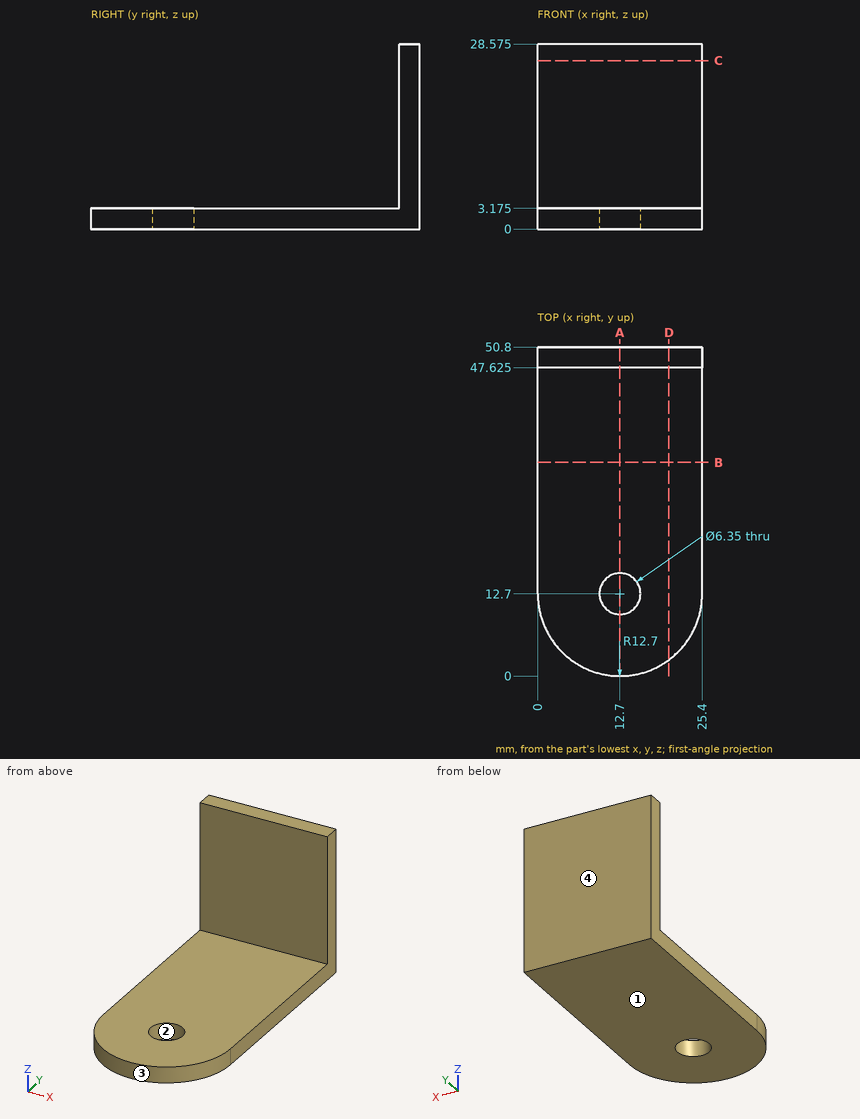
Drawing for the job (mm, zero at the part's lowest x, y, z). Round coordinates to 2 decimals unless told otherwise and drop trailing zeros. Loops run counter-clockwise (first coordinate to the right, second up) from the corner with the lowest first, then second, coordinate; pieces in that order, holes last. Notation, with made-up numbers: M 47.5,82 L 51.5,82 A27 ccw 51.5,121 Z; hole C -34,81 d7. An arc over 180 degrees is marked long. Use a Markdown table: item, result. Add a question column.
(1) Pull direction Y, two halves, no side cores. Call the marked faces 1, 2, 3 and 4: +Y half, -Y half, draft (parallel to the pull), parting line (faces both ways), or undercut.
(2) Cut at B-B (y = 33). Give the cut face in (x, z) (3 decimals), and give its area (3 significant figures).
(3) Flat gauge pins, fed straight in: pin 1 (3 mm diameter, centred on x = 7.5, y = 28, fed in from +Z) (3 decimals); pin 2 (12.5 mm diameter, centred on x = 7.5, z = 15.5, fed in from -Y) (3 decimals). Where does each tip first touch, or does it go through?
(4) Cut at C-C (z = 26). Give the cut face in (x, y) (3 decimals).
(5) Cut at A-A (x = 12.7). Give the cut face in (y, z) (3 decimals).
(6) Cut at D-D (x = 20.25). Give the cut face in (y, z) (3 decimals), and give its area (3 significant figures).
(7) Drill centre lines: line 1 (Y direction, x = 12.7, z = 2.05) (3 decimals); line 2 (Y direction, x = 18.25, z = 26) (3 decimals); line 3 (Z direction, x = 8, y = 9) (3 decimals). Where is each one in solid material? Low to high.
Geometry says:
| question | item | result |
|---|---|---|
| 1 | face 1 | draft |
| 1 | face 2 | undercut |
| 1 | face 3 | -Y half |
| 1 | face 4 | +Y half |
| 2 | outline | M 0,0 L 25.4,0 L 25.4,3.175 L 0,3.175 Z |
| 2 | area | 80.6 mm² |
| 3 | pin 1 | stops at z = 3.175 |
| 3 | pin 2 | stops at y = 47.625 |
| 4 | outline | M 0,47.625 L 25.4,47.625 L 25.4,50.8 L 0,50.8 Z |
| 5 | outline | M 0,0 L 9.525,0 L 9.525,3.175 L 0,3.175 Z; M 15.875,0 L 50.8,0 L 50.8,28.575 L 47.625,28.575 L 47.625,3.175 L 15.875,3.175 Z |
| 6 | outline | M 2.488,0 L 50.8,0 L 50.8,28.575 L 47.625,28.575 L 47.625,3.175 L 2.488,3.175 Z |
| 6 | area | 234 mm² |
| 7 | line 1 | y = 0 to 9.525, 15.875 to 50.8 |
| 7 | line 2 | y = 47.625 to 50.8 |
| 7 | line 3 | z = 0 to 3.175 |
